Could you check a few things on this model? Use its own coordinates, in mm. A direction names the side the tool comes from. Coordinates: 2 decimals unless noted, no trailing zeros. Order: outer loops, then holes, each group sorted by start corner. A loop starts at its lowest first (then second) coordinate and runs counter-clockwise, first axis right, second up. Notation, with made-up numbers: (14.25, 87.5) - (34.25, 87.5) arc R37 ccw to (34.25, 125.5) - close; hole circle Ø2 at (14, -18). An arc over 180 degrees is marked (long way). Answer as CSV lines item,"result". Start each with the question number.
1. I need wall thicknesses on probe 1 along X at (y, z) = (-44.5, 1.6); probe 2 along X at (y, z) = (0.5, 1.85); probe 3 along X at (y, z) = (-1.5, 2.9). Which ranges of each line are inside material? Lowest first, please.
2. I want a section at D-D, the plane y = 6.35. List the corners of the cut face in (x, z) for me (1 decimal), and give its area (3 significant figures).
3. I want a section at A-A, the plane y = -35. List the corners of the cut face in (x, z) for me (3 decimals), and give its area (3 significant figures).
4. For faces 1 (the face through (-9.525, -26, 2)), 2 (the face through (0, 12.7, 2)), which set-ups out of +Z, -Z, +X, -X, +Y, -Y let a thin tool reach every point of the face, with its end or its side?
5. I want a section at B-B, the plane x = 3. List the corners of the cut face in (y, z) for me (3 decimals), and give its area (3 significant figures).
6. I want a section at C-C, the plane z = 2.3. Count the separate pieces of the cut face and the enclosed holes in it, and give its area (3 significant figures).
7. For pin 1 (1.9 mm diameter, centred on x = 6.35, y = -6.35, fed in from -Z); pin 2 (1 mm diameter, centred on x = 4, z = 1.5, fed in from -Y); pin 3 (1.6 mm diameter, centred on y = -24, z = 1.5, fed in from -X); pin 4 (1 mm diameter, centred on y = -24.5, z = 1, fed in from +X), each with a flat end and sliding along its axis, tell me the tip position at first contact or that it passes through.
8. Thinking about a two-plate mould opening in X: for faces 3 (the face through (-5.09, -7.316, 1.565)), 4 (the face through (18, -22, 3.175)), 5 (the face through (31.186, 10.341, 1.565)), which applies, released by +X, released by -X, zero draft, split by the parting line, or undercut?
from build123d import *

# Parameters (mm, degrees)
SKETCH1_W                    = 19.05
SKETCH1_H                    = 25.4
BOSS_EXTRUDE1_DEPTH          = 3.175
F_3_8_CLEARANCE_HOLE1_D      = 10.0838
M12_CLEARANCE_HOLE1_D        = 13.5
F_1_8_0_125_DIAMETER_HOLE1_D = 3.175


with BuildPart() as part:
    # Sketch1 → Boss-Extrude1 (new body)
    with BuildSketch(Plane.XY):
        with BuildLine():
            Line((-23.8125, 12.7), (23.8125, 12.7))
            ThreePointArc((23.8125, 12.7), (31.276314181, 10.275284807), (35.890108891, 3.927004389))
            Line((35.890108891, 3.927004389), (51.598960291, -44.38599569))
            ThreePointArc((51.598960291, -44.38599569), (49.460825767, -54.804118571), (39.416075709, -58.298671456))
            Line((39.416075709, -58.298671456), (-10.386929216, -49.133853571))
            ThreePointArc((-10.386929216, -49.133853571), (-12.351826078, -48.282813663), (-13.745274772, -46.65696332))
            Line((-13.745274772, -46.65696332), (-35.06656606, -5.885235519))
            ThreePointArc((-35.06656606, -5.885235519), (-34.676028227, 6.578278989), (-23.8125, 12.7))
        make_face()
        with Locations((0, -25.4)):
            Rectangle(SKETCH1_W, SKETCH1_H, mode=Mode.SUBTRACT)
    extrude(amount=BOSS_EXTRUDE1_DEPTH)

    # 3/8 Clearance Hole1 (through all)
    with Locations(Plane.XY.offset(3.175)):
        with Locations((-23.8125, 0), (23.8125, 0)):
            Hole(F_3_8_CLEARANCE_HOLE1_D / 2)

    # M12 Clearance Hole1 (through all)
    with Locations(Plane.XY.offset(3.175)):
        with Locations((41.3639, -47.7139)):
            Hole(M12_CLEARANCE_HOLE1_D / 2)

    # 1/8 (0.125) Diameter Hole1 (through all)
    with Locations(Plane.XY.offset(3.175)):
        with Locations((6.35, -6.35), (-6.35, 6.35), (-6.35, -6.35), (6.35, 6.35), (-6.35, -44.45), (6.35, -44.45)):
            Hole(F_1_8_0_125_DIAMETER_HOLE1_D / 2)


solid = part.part
Solved:
1,probe 1,"x = -14.87 to -7.94, -4.76 to 4.76, 7.94 to 35.43, 47.3 to 51.64"
1,probe 2,"x = -36.5 to -28.83, -18.8 to 18.8, 28.83 to 37"
1,probe 3,"x = -36.42 to -28.63, -19 to 19, 28.63 to 37.65"
2,outline,"(-34.8, 0) - (-7.9, 0) - (-7.9, 3.2) - (-34.8, 3.2) - close; (-4.8, 0) - (4.8, 0) - (4.8, 3.2) - (-4.8, 3.2) - close; (7.9, 0) - (34.8, 0) - (34.8, 3.2) - (7.9, 3.2) - close"
2,area,"201 mm2"
3,outline,"(-19.841, 0) - (-9.525, 0) - (-9.525, 3.175) - (-19.841, 3.175) - close; (9.525, 0) - (48.547, 0) - (48.547, 3.175) - (9.525, 3.175) - close"
3,area,"157 mm2"
4,face 1,"+Z, -Z"
4,face 2,"+Z, -Z, +X, -X, +Y"
5,outline,"(-51.597, 0) - (-38.1, 0) - (-38.1, 3.175) - (-51.597, 3.175) - close; (-12.7, 0) - (12.7, 0) - (12.7, 3.175) - (-12.7, 3.175) - close"
5,area,"123 mm2"
6,separate pieces,"1"
6,enclosed holes,"10"
6,area,"3,800 mm2"
7,pin 1,"passes through"
7,pin 2,"stops at y = -51.87"
7,pin 3,"stops at x = -26.01"
7,pin 4,"stops at x = 45.3"
8,face 3,"undercut"
8,face 4,"zero draft"
8,face 5,"released by +X"
